CAD build for the part. Positions are in the model's coordinates, mm. Face numbers are marked on the shaded views. Coordinates: 2 decimals unless noted, no trailing zeros. Loops run counter-clockwise (first coordinate to the right, second up) from the corner with the lowest first, then second, coordinate; pieces in that order, holes last.
1) Wall check: line 1 along Y through (x, z) = (351, 2.5); line 2 along X through (y, z) = (-15.5, 2.8); line 3 along Y through (x, z) = (389, 3.85). Give the ranges that are in metal, low to high.
2) Saw through at B-B, the plane z = 5. Write the cut outline in (x, y), and give its area (3 significant figures).
3) Pin check, flat tips, straight feed: pin 1 Ø3 at (x, y) = (386.5, -21.5) entering from +Z; pin 2 Ø1.5 at (y, z) = (-33.5, 5) entering from +X. Stop position of each tip, or through.
4) Two-plate mould, pull along Y, no slides. Class the marked faces 1, 2 and 3: +Y half, -Y half, draft (parallel to the pull), parting line (faces both ways), or undercut.
5) Saw through at D-D, the plane y = -31.5. Write the cut outline in (x, z).
6) Saw through at A-A, the plane y = -19. Write the cut outline in (x, z), and give its area (3 significant figures).
7) Saw through at C-C, the plane x = 351.5. Write the cut outline in (y, z).
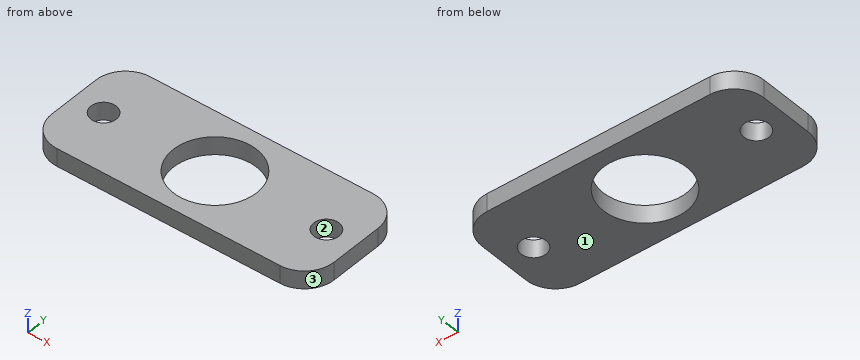
```python
from build123d import *

# Parameters (mm, degrees)
SKETCH1_W           = 95
SKETCH1_H           = 38
SKETCH1_R           = 14
SKETCH1_R_2         = 4.25
BOSS_EXTRUDE1_DEPTH = 6
FILLET1_R           = 10


with BuildPart() as part:
    # Sketch1 → Boss-Extrude1 (new body)
    with BuildSketch(Plane.XY):
        with Locations((351.5, -19)):
            Rectangle(SKETCH1_W, SKETCH1_H)
        with Locations((351.5, -19)):
            Circle(SKETCH1_R, mode=Mode.SUBTRACT)
        with Locations((389, -19)):
            Circle(SKETCH1_R_2, mode=Mode.SUBTRACT)
        with Locations(Location((314, -19, 0), (0, 0, 180))):
            Circle(SKETCH1_R_2, mode=Mode.SUBTRACT)
    extrude(amount=BOSS_EXTRUDE1_DEPTH)

    # Fillet1
    fillet1_edges = [part.edges().sort_by_distance(p)[0] for p in [
        (399, -38, 3),
        (304, -38, 3),
        (304, 0, 3),
        (399, 0, 3),
    ]]
    fillet(fillet1_edges, radius=FILLET1_R)


solid = part.part
```
Data:
1. line 1: y = -38 to -32.99, -5.01 to 0
1. line 2: x = 304 to 311.59, 316.41 to 337.94, 365.06 to 386.59, 391.41 to 399
1. line 3: y = -38 to -23.25, -14.75 to 0
2. outline: (304, -28) arc R10 ccw to (314, -38) - (389, -38) arc R10 ccw to (399, -28) - (399, -10) arc R10 ccw to (389, 0) - (314, 0) arc R10 ccw to (304, -10) - close; hole circle Ø8.5 at (314, -19); hole circle Ø28 at (351.5, -19); hole circle Ø8.5 at (389, -19)
2. area: 2,790 mm2
3. pin 1: stops at z = 6
3. pin 2: stops at x = 397.8
4. face 1: draft
4. face 2: undercut
4. face 3: -Y half
5. outline: (304.63, 0) - (345.2, 0) - (345.2, 6) - (304.63, 6) - close; (357.8, 0) - (398.37, 0) - (398.37, 6) - (357.8, 6) - close
6. outline: (304, 0) - (309.75, 0) - (309.75, 6) - (304, 6) - close; (318.25, 0) - (337.5, 0) - (337.5, 6) - (318.25, 6) - close; (365.5, 0) - (384.75, 0) - (384.75, 6) - (365.5, 6) - close; (393.25, 0) - (399, 0) - (399, 6) - (393.25, 6) - close
6. area: 300 mm2
7. outline: (-38, 0) - (-33, 0) - (-33, 6) - (-38, 6) - close; (-5, 0) - (0, 0) - (0, 6) - (-5, 6) - close
